The listing builds one solid part. Answer for the finished solid, in the listing's coordinates (mm). A direction names the side the tool comes from. Round coordinates to 2 decimals unless told otherwise and drop trailing zeros. Order: outer loops, then holes, each group sorted by start corner. A loop starts at its lowest first (then second) coordinate and runs counter-clockwise, first axis right, second up. Notation, with made-up numbers: (-22.5, -19) - (31.5, -19) arc R19 cw to (31.5, 3) - close; hole circle Ø6 at (79, 77.5). An arc over 180 degrees is marked (long way). Use CSV: the item, a comma, the result in double quotes. Start each with the question number.
Item 1: Find section B-B, the plane x = -11. Give the vertices of the cut face in (y, z), plus the area to 3 significant figures.
Item 2: Determine the mould class of faces 4 (the flat face through (-32, 15, 5)), 5 (the flat face through (35, 18, 7)), 6 (the cylindrical face through (26, 18, 7)) for opening direction X: +X half, -X half, draft (parallel to the pull), parting line (faces both ways), or undercut.
Item 3: Find section A-A, the plane z = 7. Give the vertices of the cut face in (x, y).
Item 4: Flat-ended cylindrical pins translate along their axes: P1, Ø1, axis at y = -0.5, z = 6, coming from the +X side; P2, Ø6, axis at x = 26.5, z = 9.5, coming from the -Y side; P3, Ø4, axis at y = -10, z = 11, coming from the -X side; P4, Ø5, axis at x = -29, z = 7, coming from the -Y side. Find the tip coordinate at first contact, or state that the pin passes through.
Item 5: Find section C-C, the plane z = 11. Give the vertices of the cut face in (x, y).
Item 6: Straight lines are drawn through the part: line 1 along X through (y, z) = (-3, 13); line 2 along X through (y, z) = (18, 7.75); line 3 along Z through (x, y) = (29, 19.55). For each, find the intervals that lie inside material, in ascending order. Write a range as [from, to].
Item 7: Find section D-D, the plane y = -4. Give the vertices of the cut face in (x, z).
Item 8: For faces 1 (the cylindrical face through (-14.2, -6.4, 6.9)), 2 (the flat face through (-23, -3, 7)), 3 (the flat face through (23, -3, 7)), determine the directions among +Z, -Z, +X, -X, +Y, -Y from which every point of the face is accessible in a straight line to the end or side of a thin tool.
```python
from build123d import *

# Parameters (mm, degrees)
SKETCH_1_R          = 4
SKETCH_1_R_2        = 8
EXTRUDE_1_DEPTH     = 14
SKETCH_2_R          = 3
CUT_EXTRUDE_1_DEPTH = 14


with BuildPart() as part:
    # 草图1 → 凸台-拉伸1 (new body)
    with BuildSketch(Plane.XY):
        Polygon((-35, 21), (-35, 15), (-23, 15), (-23, -21), (23, -21), (23, 15), (35, 15), (35, 21), align=None)
        with Locations((-11, -4)):
            Circle(SKETCH_1_R, mode=Mode.SUBTRACT)
        with Locations((11, -4)):
            Circle(SKETCH_1_R_2, mode=Mode.SUBTRACT)
    extrude(amount=EXTRUDE_1_DEPTH)

    # 草图2 → 切除-拉伸1 (cut)
    with BuildSketch(Plane.XZ.offset(-15)):
        with Locations((-29, 7)):
            Circle(SKETCH_2_R)
        with Locations((29, 7)):
            Circle(SKETCH_2_R)
    extrude(amount=-CUT_EXTRUDE_1_DEPTH, mode=Mode.SUBTRACT)


solid = part.part
```
Worked out:
1,outline,"(-21, 0) - (-8, 0) - (-8, 14) - (-21, 14) - close; (0, 0) - (21, 0) - (21, 14) - (0, 14) - close"
1,area,"476 mm²"
2,face 4,"draft"
2,face 5,"+X half"
2,face 6,"undercut"
3,outline,"(-35, 15) - (-32, 15) - (-32, 21) - (-35, 21) - close; (-26, 15) - (-23, 15) - (-23, -21) - (23, -21) - (23, 15) - (26, 15) - (26, 21) - (-26, 21) - close; (32, 15) - (35, 15) - (35, 21) - (32, 21) - close; hole circle Ø8 at (-11, -4); hole circle Ø16 at (11, -4)"
4,P1,"stops at x = 23"
4,P2,"stops at y = 15"
4,P3,"stops at x = -23"
4,P4,"passes through"
5,outline,"(-35, 15) - (-23, 15) - (-23, -21) - (23, -21) - (23, 15) - (35, 15) - (35, 21) - (-35, 21) - close; hole circle Ø8 at (-11, -4); hole circle Ø16 at (11, -4)"
6,line 1,"x = [-23, -14.87], [-7.13, 3.06], [18.94, 23]"
6,line 2,"x = [-35, -31.9], [-26.1, 26.1], [31.9, 35]"
6,line 3,"z = [0, 4], [10, 14]"
7,outline,"(-23, 0) - (-15, 0) - (-15, 14) - (-23, 14) - close; (-7, 0) - (3, 0) - (3, 14) - (-7, 14) - close; (19, 0) - (23, 0) - (23, 14) - (19, 14) - close"
8,face 1,"+Z, -Z"
8,face 2,"+Z, -Z, -X, -Y"
8,face 3,"+Z, -Z, +X, -Y"
